```python
from build123d import *

# Parameters (mm, degrees)
SKETCH1_W           = 42.3
SKETCH1_H           = 42.3
BOSS_EXTRUDE1_DEPTH = 48
CHAMFER1_SIZE       = 5
SKETCH2_W           = 40
SKETCH2_H           = 40
BOSS_EXTRUDE2_DEPTH = 5
CHAMFER2_SIZE       = 5
SKETCH3_R           = 18
BOSS_EXTRUDE3_DEPTH = 22.3
SKETCH4_R           = 11
BOSS_EXTRUDE4_DEPTH = 2
SKETCH5_R           = 4
BOSS_EXTRUDE5_DEPTH = 20
SKETCH6_R           = 6.210975092
BOSS_EXTRUDE6_DEPTH = 0.5
SKETCH7_R           = 1.25
CUT_EXTRUDE1_DEPTH  = 5
SKETCH8_W           = 4.27994847
SKETCH8_H           = 8.688986299
CUT_EXTRUDE2_DEPTH  = 15


with BuildPart() as part:
    # Sketch1 → Boss-Extrude1 (new body)
    with BuildSketch(Plane.XY):
        Rectangle(SKETCH1_W, SKETCH1_H)
    extrude(amount=BOSS_EXTRUDE1_DEPTH)

    # Chamfer1
    chamfer1_edges = [part.edges().sort_by_distance(p)[0] for p in [
        (21.15, -21.15, 24),
        (-21.15, -21.15, 24),
        (-21.15, 21.15, 24),
        (21.15, 21.15, 24),
    ]]
    chamfer(chamfer1_edges, length=CHAMFER1_SIZE)

    # Sketch2 → Boss-Extrude2 (add)
    with BuildSketch(Plane(origin=(0, 0, 0), x_dir=(-1, 0, 0), z_dir=(0, 0, -1))):
        Rectangle(SKETCH2_W, SKETCH2_H)
    extrude(amount=BOSS_EXTRUDE2_DEPTH)

    # Chamfer2
    # the kernel refuses this chamfer: 5 mm, written as the material it takes off along each edge
    with BuildSketch(Plane(origin=(-20, -20, 0), x_dir=(-0.027495876610586317, 0.9996219169112968, 0), z_dir=(0, 0, -1)), Plane(origin=(-20, 20, 0), x_dir=(0.9996219169112968, 0.027495876610586317, 0), z_dir=(0, 0, -1))) as chamfer2_piece_1:
        Polygon((CHAMFER2_SIZE * 0.999621916911, CHAMFER2_SIZE * 0.0274958766106), (-CHAMFER2_SIZE * 0.0274958766106, CHAMFER2_SIZE * 0.999621916911), (0, 0), align=None)
    extrude(amount=17.85841494, mode=Mode.SUBTRACT)
    with BuildSketch(Plane(origin=(20, 20, 0), x_dir=(-0.9996219169112968, 0.027495876610586317, 0), z_dir=(0, 0, -1)), Plane(origin=(20, -20, 0), x_dir=(0.027495876610586317, 0.9996219169112968, 0), z_dir=(0, 0, -1))) as chamfer2_piece_2:
        Polygon((CHAMFER2_SIZE * 0.999621916911, -CHAMFER2_SIZE * 0.0274958766106), (-CHAMFER2_SIZE * 0.0274958766106, -CHAMFER2_SIZE * 0.999621916911), (0, 0), align=None)
    extrude(amount=17.85841494, mode=Mode.SUBTRACT)

    # Sketch3 → Boss-Extrude3 (add)
    with BuildSketch(Plane(origin=(0, 0, -5), x_dir=(-1, 0, 0), z_dir=(0, 0, -1))):
        with Locations(Location((0, 0, 0), (0, 0, 180))):
            Circle(SKETCH3_R)
    extrude(amount=BOSS_EXTRUDE3_DEPTH)

    # Sketch4 → Boss-Extrude4 (add)
    with BuildSketch(Plane(origin=(0, 0, -27.3), x_dir=(-1, 0, 0), z_dir=(0, 0, -1))):
        Circle(SKETCH4_R)
    extrude(amount=BOSS_EXTRUDE4_DEPTH)

    # Sketch5 → Boss-Extrude5 (add)
    with BuildSketch(Plane(origin=(0, 0, -29.3), x_dir=(-1, 0, 0), z_dir=(0, 0, -1))):
        Circle(SKETCH5_R)
    extrude(amount=BOSS_EXTRUDE5_DEPTH)

    # Sketch6 → Boss-Extrude6 (add)
    with BuildSketch(Plane(origin=(0, 0, -29.3), x_dir=(-1, 0, 0), z_dir=(0, 0, -1))):
        Circle(SKETCH6_R)
    extrude(amount=BOSS_EXTRUDE6_DEPTH)

    # Sketch7 → Cut-Extrude1 (cut)
    with BuildSketch(Plane(origin=(0, 0, -27.3), x_dir=(-1, 0, 0), z_dir=(0, 0, -1))):
        with Locations((9.899494937, 9.899494937)):
            Circle(SKETCH7_R)
        with Locations((9.899494937, -9.899494937)):
            Circle(SKETCH7_R)
        with Locations((-9.899494937, -9.899494937)):
            Circle(SKETCH7_R)
        with Locations((-9.899494937, 9.899494937)):
            Circle(SKETCH7_R)
    extrude(amount=-CUT_EXTRUDE1_DEPTH, mode=Mode.SUBTRACT)

    # Sketch8 → Cut-Extrude2 (cut)
    with BuildSketch(Plane(origin=(0, 0, -49.3), x_dir=(-1, 0, 0), z_dir=(0, 0, -1))):
        with Locations((5.139974235, -0.230171823)):
            Rectangle(SKETCH8_W, SKETCH8_H)
    extrude(amount=-CUT_EXTRUDE2_DEPTH, mode=Mode.SUBTRACT)


solid = part.part
```
Could you check a few things on this model? Use its own coordinates, in mm. A direction names the side the tool comes from. Give positions to 0.01 mm unless a question says otherwise; leave off trailing zeros. Order: outer loops, then holes, each group sorted by start corner. A loop starts at its lowest first (then second) coordinate and runs counter-clockwise, first axis right, second up.
Q1. If I drill on line 1 along Z through (x, y) = (10, 7); line 2 along Z through (x, y) = (18.5, -8.5); line 3 along Y through (x, z) = (9, -2), over which ranges is the centre line in solid material (lowest first)?
Q2. For faces 4 (the flat face through (10, -10, -22.3)), 5 (the flat face through (0, -20, -2)), 6 (the flat face through (20, 0, -2)), 7 (the flat face through (0, 20, -2)), 8 (the flat face through (-18, -17, -2)), which set-ups out of +Z, -Z, +X, -X, +Y, -Y let a thin tool reach every point of the face, with its end or its side?
Q3. I'm going to push flat-ended pins straight in: P1, Ø10, axis at y = -8, z = -16, coming from the +X side; P2, Ø12.5, axis at x = 6.5, y = -8, coming from the -Z side; P3, Ø1.6, axis at y = 0, z = -40.5, coming from the -X side. Where does each tip first touch, or does it pass through?
Q4. We'd pull the mould along X, two halves only. Please class faces 1 (the flat face through (-8, 8, -27.3)), 2 (the flat face through (-18.6, 18.7, 23.7)), 3 (the flat face through (-10, -10, -22.3)): +X half, -X half, draft (parallel to the pull), parting line (faces both ways), or undercut.
Q5. Suppose I cut it at A-A, the plane y = 0. Write out the boundary of the cut face in (x, z), and give its area (3 significant figures).
Q6. Suppose I cut it at C-C, the plane x = 0. Write out the boundary of the cut face in (y, z), and give its area (3 significant figures).
Q7. Suppose I cut it at D-D, the plane z = -20.5. Write out the boundary of the cut face in (x, y), and give its area (3 significant figures).
Q8. Suppose I cut it at B-B, the plane z = 17. Write out the boundary of the cut face in (x, y), and give its area (3 significant figures).
Solution:
1. line 1: z = -27.3 to 48
1. line 2: z = -5 to 48
1. line 3: y = -20 to 20
2. face 4: -Z
2. face 5: -Z, +X, -X, -Y
2. face 6: -Z, +X, +Y, -Y
2. face 7: -Z, +X, -X, +Y
2. face 8: -Z, -X, -Y
3. P1: stops at x = 17.75
3. P2: stops at z = -29.8
3. P3: stops at x = -3
4. face 1: draft
4. face 2: -X half
4. face 3: undercut
5. outline: (-21.15, 0) - (-20, 0) - (-20, -5) - (-18, -5) - (-18, -27.3) - (-11, -27.3) - (-11, -29.3) - (-6.21, -29.3) - (-6.21, -29.8) - (-4, -29.8) - (-4, -34.3) - (-3, -34.3) - (-3, -49.3) - (4, -49.3) - (4, -29.8) - (6.21, -29.8) - (6.21, -29.3) - (11, -29.3) - (11, -27.3) - (18, -27.3) - (18, -5) - (20, -5) - (20, 0) - (21.15, 0) - (21.15, 48) - (-21.15, 48) - close
5. area: 3,220 mm2
6. outline: (-21.15, 0) - (-20, 0) - (-20, -5) - (-18, -5) - (-18, -27.3) - (-11, -27.3) - (-11, -29.3) - (-6.21, -29.3) - (-6.21, -29.8) - (-4, -29.8) - (-4, -49.3) - (4, -49.3) - (4, -29.8) - (6.21, -29.8) - (6.21, -29.3) - (11, -29.3) - (11, -27.3) - (18, -27.3) - (18, -5) - (20, -5) - (20, 0) - (21.15, 0) - (21.15, 48) - (-21.15, 48) - close
6. area: 3,240 mm2
7. outline: circle Ø36 at (0, 0)
7. area: 1,020 mm2
8. outline: (-21.15, -16.15) - (-16.15, -21.15) - (16.15, -21.15) - (21.15, -16.15) - (21.15, 16.15) - (16.15, 21.15) - (-16.15, 21.15) - (-21.15, 16.15) - close
8. area: 1,740 mm2
